from build123d import *
from OCP.BRepFilletAPI import BRepFilletAPI_MakeChamfer

# Parameters (mm, degrees)
SKETCH_1_W           = 40
SKETCH_1_H           = 20
SKETCH_1_R           = 1.55
SKETCH_1_W_2         = 20
SKETCH_1_H_2         = 10
EXTRUDE_1_DEPTH      = 3
SKETCH_2_R           = 2
EXTRUDE_2_DEPTH      = 3
FILLET_1_R           = 2
SKETCH_3_W           = 10
SKETCH_3_H           = 10
CUT_EXTRUDE_1_DEPTH  = 33.155870382
CHAMFER_1_SIZE       = 6
CHAMFER_1_SIZE_2     = 10
FILLET_2_OUTLINE_R   = 2
FILLET_2_OUTLINE_R_2 = 1.55
FILLET_2_OUTLINE_W   = 20
FILLET_2_OUTLINE_H   = 10
FILLET_2_DEPTH       = 3
CUT_EXTRUDE_2_DEPTH  = 33.155870382
SKETCH_5_R           = 2
EXTRUDE_3_DEPTH      = 3
FILLET_3_R           = 1
SKETCH_6_R           = 2
EXTRUDE_4_DEPTH      = 3
SKETCH_7_R           = 2
CUT_EXTRUDE_3_DEPTH  = 33.155870382


with BuildPart() as part:
    # 草图1 → 凸台-拉伸1 (new body)
    with BuildSketch(Plane(origin=(0, 0, 0), x_dir=(1, 0, 0), z_dir=(0, 1, 0))):
        Rectangle(SKETCH_1_W, SKETCH_1_H)
        with Locations(Location((-16, 6, 0), (0, 0, 270))):
            Circle(SKETCH_1_R, mode=Mode.SUBTRACT)
        with Locations(Location((16, 6, 0), (0, 0, 90))):
            Circle(SKETCH_1_R, mode=Mode.SUBTRACT)
        with Locations(Location((16, -6, 0), (0, 0, 270))):
            Circle(SKETCH_1_R, mode=Mode.SUBTRACT)
        with Locations(Location((-16, -6, 0), (0, 0, 90))):
            Circle(SKETCH_1_R, mode=Mode.SUBTRACT)
        Rectangle(SKETCH_1_W_2, SKETCH_1_H_2, mode=Mode.SUBTRACT)
    extrude(amount=EXTRUDE_1_DEPTH)

    # 草图2 → 凸台-拉伸2 (add, through all)
    with BuildSketch(Plane(origin=(0, 3, 0), x_dir=(1, 0, 0), z_dir=(0, 1, 0))):
        with BuildLine():
            Line((-8.17, 20), (-8.17, -20))
            ThreePointArc((-8.17, -20), (-3.17, -25), (1.83, -20))
            Line((1.83, -20), (1.83, 20))
            ThreePointArc((1.83, 20), (-3.17, 25), (-8.17, 20))
        make_face()
        with Locations(Location((-3.17, 20, 0), (0, 0, 270))):
            Circle(SKETCH_2_R, mode=Mode.SUBTRACT)
        with Locations(Location((-3.17, -20, 0), (0, 0, 270))):
            Circle(SKETCH_2_R, mode=Mode.SUBTRACT)
    extrude(amount=-EXTRUDE_2_DEPTH)

    # 圆角1
    fillet_1_edges = [part.edges().sort_by_distance(p)[0] for p in [
        (20, 1.5, 10),
        (-20, 1.5, 10),
        (-20, 1.5, -10),
        (20, 1.5, -10),
    ]]
    fillet(fillet_1_edges, radius=FILLET_1_R)

    # 草图3 → 切除-拉伸1 (cut, through all)
    with BuildSketch(Plane(origin=(0, 3, 0), x_dir=(1, 0, 0), z_dir=(0, 1, 0))):
        with Locations((-3.17, 0)):
            Rectangle(SKETCH_3_W, SKETCH_3_H)
    extrude(amount=-CUT_EXTRUDE_1_DEPTH, mode=Mode.SUBTRACT)

    # 倒角1
    chamfer_1_edges_1 = [part.edges().sort_by_distance(p)[0] for p in [
        (-8.17, 1.5, 10),
    ]]
    chamfer_1_side_1 = [part.faces().sort_by_distance(p)[0] for p in [
        (-8.29, 1.5, 10),
    ]]
    chamfer_1_edges_2 = [part.edges().sort_by_distance(p)[0] for p in [
        (1.83, 1.5, 10),
    ]]
    chamfer_1_side_2 = [part.faces().sort_by_distance(p)[0] for p in [
        (1.95, 1.5, 10),
    ]]
    chamfer_1_edges_3 = [part.edges().sort_by_distance(p)[0] for p in [
        (1.83, 1.5, -10),
    ]]
    chamfer_1_side_3 = [part.faces().sort_by_distance(p)[0] for p in [
        (1.83, 1.5, -10.12),
    ]]
    chamfer_1_edges_4 = [part.edges().sort_by_distance(p)[0] for p in [
        (-8.17, 1.5, -10),
    ]]
    chamfer_1_side_4 = [part.faces().sort_by_distance(p)[0] for p in [
        (-8.29, 1.5, -10),
    ]]
    chamfer_1 = BRepFilletAPI_MakeChamfer(part.part.solid().wrapped)
    for e in chamfer_1_edges_1:
        chamfer_1.Add(CHAMFER_1_SIZE - 0.0001, CHAMFER_1_SIZE_2 - 0.0001, e.wrapped, chamfer_1_side_1[0].wrapped)
    for e in chamfer_1_edges_2:
        chamfer_1.Add(CHAMFER_1_SIZE - 0.0001, CHAMFER_1_SIZE_2 - 0.0001, e.wrapped, chamfer_1_side_2[0].wrapped)
    for e in chamfer_1_edges_3:
        chamfer_1.Add(CHAMFER_1_SIZE_2 - 0.0001, CHAMFER_1_SIZE - 0.0001, e.wrapped, chamfer_1_side_3[0].wrapped)
    for e in chamfer_1_edges_4:
        chamfer_1.Add(CHAMFER_1_SIZE - 0.0001, CHAMFER_1_SIZE_2 - 0.0001, e.wrapped, chamfer_1_side_4[0].wrapped)
    add(Compound.cast(chamfer_1.Shape()), mode=Mode.REPLACE)  # a hair under: the kernel refuses the full size

    # 圆角2: read off the stored shape, not the designer's step
    # 圆角2 outline → 圆角2 (add)
    with BuildSketch(Plane(origin=(0, 0, 0), x_dir=(1, 0, 0), z_dir=(0, 1, 0))):
        with BuildLine():
            ThreePointArc((18, -10), (19.414213562, -9.414213562), (20, -8))
            Line((20, -8), (20, 8))
            ThreePointArc((20, 8), (19.414213562, 9.414213562), (18, 10))
            Line((18, 10), (9.528571137, 10))
            ThreePointArc((9.528571137, 10), (8.050474692, 10.38940028), (6.95609236, 11.456512734))
            Line((6.95609236, 11.456512734), (2.204529459, 19.375784235))
            ThreePointArc((2.204529459, 19.375784235), (1.9367411, 19.953413027), (1.796880148, 20.574544688))
            ThreePointArc((1.796880148, 20.574544688), (-3.17, 25), (-8.136880148, 20.574544688))
            ThreePointArc((-8.136880148, 20.574544688), (-8.2767411, 19.953413027), (-8.544529459, 19.375784235))
            Line((-8.544529459, 19.375784235), (-13.29609236, 11.456512734))
            ThreePointArc((-13.29609236, 11.456512734), (-14.390474692, 10.38940028), (-15.868571137, 10))
            Line((-15.868571137, 10), (-18, 10))
            ThreePointArc((-18, 10), (-19.414213562, 9.414213562), (-20, 8))
            Line((-20, 8), (-20, -8))
            ThreePointArc((-20, -8), (-19.414213562, -9.414213562), (-18, -10))
            Line((-18, -10), (-15.868571137, -10))
            ThreePointArc((-15.868571137, -10), (-14.390474692, -10.38940028), (-13.29609236, -11.456512734))
            Line((-13.29609236, -11.456512734), (-8.544529459, -19.375784235))
            ThreePointArc((-8.544529459, -19.375784235), (-8.2767411, -19.953413027), (-8.136880148, -20.574544688))
            ThreePointArc((-8.136880148, -20.574544688), (-3.17, -25), (1.796880148, -20.574544688))
            ThreePointArc((1.796880148, -20.574544688), (1.9367411, -19.953413027), (2.204529459, -19.375784235))
            Line((2.204529459, -19.375784235), (6.95609236, -11.456512734))
            ThreePointArc((6.95609236, -11.456512734), (8.050474692, -10.38940028), (9.528571137, -10))
            Line((9.528571137, -10), (18, -10))
        make_face()
        with Locations((-3.17, -20)):
            Circle(FILLET_2_OUTLINE_R, mode=Mode.SUBTRACT)
        with Locations((-16, -6)):
            Circle(FILLET_2_OUTLINE_R_2, mode=Mode.SUBTRACT)
        with Locations((16, -6)):
            Circle(FILLET_2_OUTLINE_R_2, mode=Mode.SUBTRACT)
        with Locations((-16, 6)):
            Circle(FILLET_2_OUTLINE_R_2, mode=Mode.SUBTRACT)
        with Locations((-3.17, 20)):
            Circle(FILLET_2_OUTLINE_R, mode=Mode.SUBTRACT)
        Rectangle(FILLET_2_OUTLINE_W, FILLET_2_OUTLINE_H, mode=Mode.SUBTRACT)
        with Locations((16, 6)):
            Circle(FILLET_2_OUTLINE_R_2, mode=Mode.SUBTRACT)
    extrude(amount=FILLET_2_DEPTH)

    # 草图4 → 切除-拉伸2 (cut, through all)
    with BuildSketch(Plane(origin=(0, 3, 0), x_dir=(1, 0, 0), z_dir=(0, 1, 0))):
        Polygon((-10, 5), (-4, 15), (0, 15), (6, 5), align=None)
        Polygon((-10, -5), (6, -5), (0, -15), (-4, -15), align=None)
    extrude(amount=-CUT_EXTRUDE_2_DEPTH, mode=Mode.SUBTRACT)

    # 草图5 → 凸台-拉伸3 (add, through all)
    with BuildSketch(Plane(origin=(0, 3, 0), x_dir=(1, 0, 0), z_dir=(0, 1, 0))):
        with BuildLine():
            Line((-10, 1.5), (-5.912088761, 4.18102251))
            ThreePointArc((-5.912088761, 4.18102251), (-5.06302182, 4.627793036), (-4.144252411, 4.904164785))
            Line((-4.144252411, 4.904164785), (4.971008489, 6.714985851))
            Line((4.971008489, 6.714985851), (6, 5))
            Line((6, 5), (1.83, 0))
            Line((1.83, 0), (6, -5))
            Line((6, -5), (4.971008489, -6.714985851))
            Line((4.971008489, -6.714985851), (-4.144252411, -4.904164785))
            ThreePointArc((-4.144252411, -4.904164785), (-5.06302182, -4.627793036), (-5.912088761, -4.18102251))
            Line((-5.912088761, -4.18102251), (-10, -1.5))
            Line((-10, -1.5), (-10, 1.5))
        make_face()
        with Locations(Location((-3.17, 0, 0), (0, 0, 270))):
            Circle(SKETCH_5_R, mode=Mode.SUBTRACT)
    extrude(amount=-EXTRUDE_3_DEPTH)

    # 圆角3
    fillet_3_edges = [part.edges().sort_by_distance(p)[0] for p in [
        (6, 1.5, -5),
        (-4, 1.5, -15),
        (0, 1.5, -15),
        (-4, 1.5, 15),
        (6, 1.5, 5),
        (0, 1.5, 15),
        (-10, 1.5, 1.5),
        (-10, 1.5, -1.5),
        (4.971008489, 1.5, -6.714985851),
        (1.83, 1.5, 0),
        (4.971008489, 1.5, 6.714985851),
        (10, 1.5, 5),
        (10, 1.5, -5),
        (-10, 1.5, -5),
        (-10, 1.5, 5),
    ]]
    fillet(fillet_3_edges, radius=FILLET_3_R)

    # 草图6 → 凸台-拉伸4 (add, through all)
    with BuildSketch(Plane(origin=(0, 3, 0), x_dir=(1, 0, 0), z_dir=(0, 1, 0))):
        with Locations((-3.17, -20)):
            Circle(SKETCH_6_R)
        with Locations((-3.17, 0)):
            Circle(SKETCH_6_R)
        with Locations((-3.17, 20)):
            Circle(SKETCH_6_R)
    extrude(amount=-EXTRUDE_4_DEPTH)

    # 草图7 → 切除-拉伸3 (cut, through all)
    with BuildSketch(Plane(origin=(0, 3, 0), x_dir=(1, 0, 0), z_dir=(0, 1, 0))):
        with Locations(Location((-3.175, 20, 0), (0, 0, 270))):
            Circle(SKETCH_7_R)
        with Locations(Location((-3.175, 0, 0), (0, 0, 270))):
            Circle(SKETCH_7_R)
        with Locations(Location((-3.175, -20, 0), (0, 0, 270))):
            Circle(SKETCH_7_R)
    extrude(amount=-CUT_EXTRUDE_3_DEPTH, mode=Mode.SUBTRACT)


solid = part.part
Geometry check sheet. Reference: the model listing, model coordinates, mm. A direction names the side the tool comes from. Coordinates: 2 decimals unless noted, no trailing zeros. Loops run counter-clockwise (first coordinate to the right, second up) from the corner with the lowest first, then second, coordinate; pieces in that order, holes last. Notation, with made-up numbers: (71.25, -23) - (121.25, -23) arc R4 ccw to (121.25, -16) - close; hole circle Ø11 at (-34.5, 51). An arc over 180 degrees is marked (long way). Use one line per item in the form item = value. Start each with the question number.
Item 1: Section check D-D, the plane x = 5. Enter the section's corners in (y, z).
Item 2: Section check B-B, the plane x = 16. Enter the section's corners in (y, z).
Item 3: Section check C-C, the plane z = 0. Enter the section's corners in (x, y) (3 decimals).
Item 4: Thickness scan on probe 1 along Z at (x, y) = (-6, 0.35); probe 2 along Z at (x, y) = (-5.5, 0.25); probe 3 along Z at (x, y) = (-4, 0.6). Record the ranges inside material, lowest first.
Item 5: Tool access check on faces 1 (the face through (4.29, 1.48, 7)), 2 (the face through (8.03, 1.48, 10.4)). Record the directions out of +Z, -Z, +X, -X, +Y, -Y that give a thin tool (end or side, any length) a straight path to the whole face; none if there is none.
Item 6: Section check A-A, the plane z = 12. Enter the section's corners in (x, y).
Item 7: Mould release check, pull along Z, two halves, no side actions. Record for faces 3 (the face through (-9.462, 1.479, -2.465)), 4 (the face through (4.55, 1.48, 15.47)), 5 (the face through (14, 1, -10)): +Z half, -Z half, draft (parallel to the pull), parting line (faces both ways), or undercut.
Item 8: Gauge pin test, flat ends, axial feed: pin 1 (8 mm diameter, centred on x = 1, z = -17.5, fed in from -Y); pin 2 (1.5 mm diameter, centred on y = 1.5, z = 16, fed in from -X); pin 3 (0.9 mm diameter, centred on x = 12, y = 2, fed in from +Z); pin 4 (1.7 mm diameter, centred on x = -17.5, y = 1.5, fed in from -Z). Record the tip position at first contact, or that the pin passes through.
Computed:
q1.outline = (0, -14.72) - (3, -14.72) - (3, -3.8) - (0, -3.8) - close; (0, 3.8) - (3, 3.8) - (3, 14.72) - (0, 14.72) - close
q2.outline = (0, -10) - (3, -10) - (3, -7.55) - (0, -7.55) - close; (0, -4.45) - (3, -4.45) - (3, 4.45) - (0, 4.45) - close; (0, 7.55) - (3, 7.55) - (3, 10) - (0, 10) - close
q3.outline = (-20, 0) - (-5.175, 0) - (-5.175, 3) - (-20, 3) - close; (-1.175, 0) - (2.132, 0) - (2.132, 3) - (-1.175, 3) - close; (10, 0) - (20, 0) - (20, 3) - (10, 3) - close
q4.probe_1 = -24.12 to -11.67, -4.12 to 4.12, 11.67 to 24.12
q4.probe_2 = -24.42 to -12.5, -4.42 to 4.42, 12.5 to 24.42
q4.probe_3 = -24.93 to -21.82, -18.18 to -14.82, -4.93 to -1.82, 1.82 to 4.93, 14.82 to 18.18, 21.82 to 24.93
q5.face_1 = +Y, -Y
q5.face_2 = +Z, +X, +Y, -Y
q6.outline = (-12.97, 0) - (-5.8, 0) - (-5.8, 3) - (-12.97, 3) - close; (1.8, 0) - (6.63, 0) - (6.63, 3) - (1.8, 3) - close
q7.face_3 = undercut
q7.face_4 = +Z half
q7.face_5 = -Z half
q8.pin_1 = 0
q8.pin_2 = -11.02
q8.pin_3 = 10
q8.pin_4 = -10
